from build123d import *

# Parameters (mm, degrees)
SKETCH_R     = 6.5
PAD_DEPTH    = 1.5
SKETCH001_R  = 5.292227
PAD001_DEPTH = 4.5
FILLET_R     = 1
FILLET001_R  = 0.3
SKETCH002_W  = 6
SKETCH002_H  = 5.5
PAD002_DEPTH = 2.5


with BuildPart() as part:
    # Sketch → Pad (new body)
    with BuildSketch(Plane.XY):
        Circle(SKETCH_R)
    extrude(amount=PAD_DEPTH)

    # Sketch001 → Pad001 (new body)
    with BuildSketch(Plane.XY.offset(1.5)):
        Circle(SKETCH001_R)
    extrude(amount=PAD001_DEPTH)

    # Fillet
    fillet_edges = [part.edges().sort_by_distance(p)[0] for p in [
        (-5.292227, 0, 6),
    ]]
    fillet(fillet_edges, radius=FILLET_R)

    # Fillet001
    fillet001_edges = [part.edges().sort_by_distance(p)[0] for p in [
        (-6.5, 0, 1.5),
    ]]
    fillet(fillet001_edges, radius=FILLET001_R)

    # Sketch002 → Pad002 (new body)
    with BuildSketch(Plane(origin=(0, 0, 0), x_dir=(1, 0, 0), z_dir=(0, 0, -1))):
        Rectangle(SKETCH002_W, SKETCH002_H)
    extrude(amount=PAD002_DEPTH)


solid = part.part
Here's how the part is built. I have some questions about the finished solid (model axes, mm). A direction names the side the tool comes from. Give positions to 0.01 mm unless a question says otherwise; leave off trailing zeros. Order: outer loops, then holes, each group sorted by start corner. A loop starts at its lowest first (then second) coordinate and runs counter-clockwise, first axis right, second up. Notation, with made-up numbers: (5.5, 89.25) -> (15.5, 89.25) arc R30 ccw to (15.5, 126.25) -> close; hole circle Ø4 at (65, -28.75). An arc over 180 degrees is marked (long way). Use a Markdown table: item, result. Add a question column.
Item 1: I need wall thicknesses on line 1 (X direction, y = -2.25, z = -0.25); line 2 (Z direction, x = 4.25, y = 3.25); line 3 (Y direction, x = -1, z = -0.5). Which ranges of each line are inside material? Lowest first, please.
Item 2: For faces 1 (the face through (-0.689, 5.247, 3.226)), 2 (the face through (0, -2.75, -1)), 3 (the face through (0, 2.75, -1)), 4 (the face through (-3, 0, -1)), which set-ups out of +Z, -Z, +X, -X, +Y, -Y let a thin tool reach every point of the face, with its end or its side?
Item 3: Imagine slicing it at C-C on z = 4. Please give me the cut outline in (x, y).
Item 4: Imagine slicing it at A-A on y = 0. Please give me the cut outline in (x, z).
Item 5: Imagine slicing it at B-B on x = 0. Please give me the cut outline in (y, z), plus the area to 3 significant figures.
Item 6: Will these pins go through, and if not, where does the flat tip stop? pin 1 (1 mm diameter, centred on x = -1, y = -5, fed in from +Z); pin 2 (1.2 mm diameter, centred on x = 1.5, z = -1.5, fed in from +Y); pin 3 (5 mm diameter, centred on x = 3, z = 0, fed in from +Y).
Data:
| question | item | result |
|---|---|---|
| 1 | line 1 | x = -3 to 3 |
| 1 | line 2 | z = 0 to 1.5 |
| 1 | line 3 | y = -2.75 to 2.75 |
| 2 | face 1 | +Z |
| 2 | face 2 | -Z, +X, -X, -Y |
| 2 | face 3 | -Z, +X, -X, +Y |
| 2 | face 4 | -Z, -X, +Y, -Y |
| 3 | outline | circle Ø10.58 at (0, 0) |
| 4 | outline | (-6.5, 0) -> (-3, 0) -> (-3, -2.5) -> (3, -2.5) -> (3, 0) -> (6.5, 0) -> (6.5, 1.2) arc R0.3 ccw to (6.2, 1.5) -> (5.29, 1.5) -> (5.29, 5) arc R1 ccw to (4.29, 6) -> (-4.29, 6) arc R1 ccw to (-5.29, 5) -> (-5.29, 1.5) -> (-6.2, 1.5) arc R0.3 ccw to (-6.5, 1.2) -> close |
| 5 | outline | (-6.5, 0) -> (-2.75, 0) -> (-2.75, -2.5) -> (2.75, -2.5) -> (2.75, 0) -> (6.5, 0) -> (6.5, 1.2) arc R0.3 ccw to (6.2, 1.5) -> (5.29, 1.5) -> (5.29, 5) arc R1 ccw to (4.29, 6) -> (-4.29, 6) arc R1 ccw to (-5.29, 5) -> (-5.29, 1.5) -> (-6.2, 1.5) arc R0.3 ccw to (-6.5, 1.2) -> close |
| 5 | area | 80.4 mm² |
| 6 | pin 1 | stops at z = 5.95 |
| 6 | pin 2 | stops at y = 2.75 |
| 6 | pin 3 | stops at y = 6.48 |
